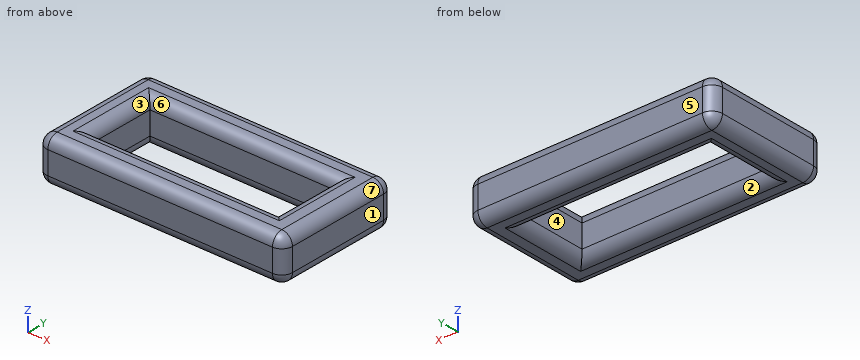
```python
from build123d import *

# Parameters (mm, degrees)
F0_W     = 117
F0_H     = 60
F0_W_2   = 88.02
F0_H_2   = 31.22
F1_DEPTH = 21
F2_R     = 5.08


with BuildPart() as f1:
    # F0 (on Top) → F1 (new body)
    with BuildSketch(Plane.XY):
        with Locations((1.678534, 44.450285)):
            Rectangle(F0_W, F0_H)
        with Locations((1.188534, 44.450285)):
            Rectangle(F0_W_2, F0_H_2, mode=Mode.SUBTRACT)
    extrude(amount=-F1_DEPTH)

    # F2
    f2_edges = [f1.edges().sort_by_distance(p)[0] for p in [
        (-56.821466, 44.450285, 0),
        (1.678534, 14.450285, 0),
        (60.178534, 44.450285, 0),
        (1.678534, 74.450285, 0),
        (1.678534, 14.450285, -21),
        (60.178534, 44.450285, -21),
        (1.678534, 74.450285, -21),
        (-56.821466, 44.450285, -21),
        (-56.821466, 14.450285, -10.5),
        (-56.821466, 74.450285, -10.5),
        (60.178534, 14.450285, -10.5),
        (60.178534, 74.450285, -10.5),
        (45.198534, 44.450285, -21),
        (1.188534, 60.060285, -21),
        (-42.821466, 44.450285, -21),
        (1.188534, 28.840285, -21),
        (1.188534, 28.840285, 0),
        (-42.821466, 44.450285, 0),
        (45.198534, 44.450285, 0),
        (1.188534, 60.060285, 0),
    ]]
    fillet(f2_edges, radius=F2_R)


solid = f1.part
```
Model file for the job. Use its own axes, mm. Face numbers are marked on the shaded views. A direction names the side the tool comes from. Give positions to 0.01 mm unless a question says otherwise; leave off trailing zeros. Loops run counter-clockwise (first coordinate to the right, second up) from the corner with the lowest first, then second, coordinate; pieces in that order, holes last. Notation, with made-up numbers: M 83,72.25 L 126,72.25 A33 ccw 126,111.25 Z; hole C 65,-22 d6. An arc over 180 degrees is marked long. Use one line per item in the form item = value.
Item 1: Slice it at B-B on x = 43. List the corners of the cut face in (y, z), and give its area (3 significant figures).
Filled in:
outline = M 14.45,-15.92 A5.08 ccw 19.53,-21 L 23.76,-21 A5.08 ccw 28.84,-15.92 L 28.84,-5.08 A5.08 ccw 23.76,0 L 19.53,0 A5.08 ccw 14.45,-5.08 Z; M 60.06,-15.92 A5.08 ccw 65.14,-21 L 69.37,-21 A5.08 ccw 74.45,-15.92 L 74.45,-5.08 A5.08 ccw 69.37,0 L 65.14,0 A5.08 ccw 60.06,-5.08 Z
area = 560 mm^2
Item 2: Slice it at A-A on y = 53. List the corners of the cut face in (x, z), and give its area (3 significant figures).
Filled in:
outline = M -56.82,-15.92 A5.08 ccw -51.74,-21 L -47.9,-21 A5.08 ccw -42.82,-15.92 L -42.82,-5.08 A5.08 ccw -47.9,0 L -51.74,0 A5.08 ccw -56.82,-5.08 Z; M 45.2,-15.92 A5.08 ccw 50.28,-21 L 55.1,-21 A5.08 ccw 60.18,-15.92 L 60.18,-5.08 A5.08 ccw 55.1,0 L 50.28,0 A5.08 ccw 45.2,-5.08 Z
area = 564 mm^2
Item 3: Which spindle directions (+Z, -Z, +X, -X, +Y, -Y) get a long thin tool onto all of the face, cutting with end or side? Do the marked faces 1, 2, 3 and 4. Say none if no direction does.
Filled in:
face_1 = +Z, -Z, +X, +Y, -Y
face_2 = -Z
face_3 = +Z
face_4 = +Z, -Z
Item 4: Slice it at C-C on z = -11.5. List the corners of the cut face in (x, y).
Filled in:
outline = M -56.82,19.53 A5.08 ccw -51.74,14.45 L 55.1,14.45 A5.08 ccw 60.18,19.53 L 60.18,69.37 A5.08 ccw 55.1,74.45 L -51.74,74.45 A5.08 ccw -56.82,69.37 Z; hole M -42.82,28.84 L 45.2,28.84 L 45.2,60.06 L -42.82,60.06 Z
Item 5: Flat gauge pins, fed straight in: pin 1 Ø6 at (x, y) = (-24.5, 57.5) entering from -Z; pin 2 Ø4 at (y, z) = (30.5, -19) entering from +X; pin 3 Ø2 at (x, z) = (-44, -3.5) entering from +Y. Where does each tip first touch, or does it go through?
Filled in:
pin_1 = -17.99
pin_2 = 60.06
pin_3 = 74.42
Item 6: Two-plate mould, pull along X, no slides. Class the marked faces 5, 6 and 7: released by +X, released by -X, zero draft, split by the parting line, or undercut.
Filled in:
face_5 = zero draft
face_6 = undercut
face_7 = released by +X
Item 7: Drill centre lines: L1, parallel to Y at x = 38, z = -11; L2, parallel to X at y = 43, z = -8.5; L3, parallel to Y at x = -19.5, z = -3.25. Where is each one in solid material? Low to high.
Filled in:
L1 = 14.45 to 28.84, 60.06 to 74.45
L2 = -56.82 to -42.82, 45.2 to 60.18
L3 = 14.79 to 28.5, 60.4 to 74.11
Item 8: Slice it at D-D on y = 70.5. List the corners of the cut face in (x, z).
Filled in:
outline = M -56.69,-15.92 A4.95 ccw -51.74,-20.87 L 55.1,-20.87 A4.95 ccw 60.05,-15.92 L 60.05,-5.08 A4.95 ccw 55.1,-0.13 L -51.74,-0.13 A4.95 ccw -56.69,-5.08 Z
